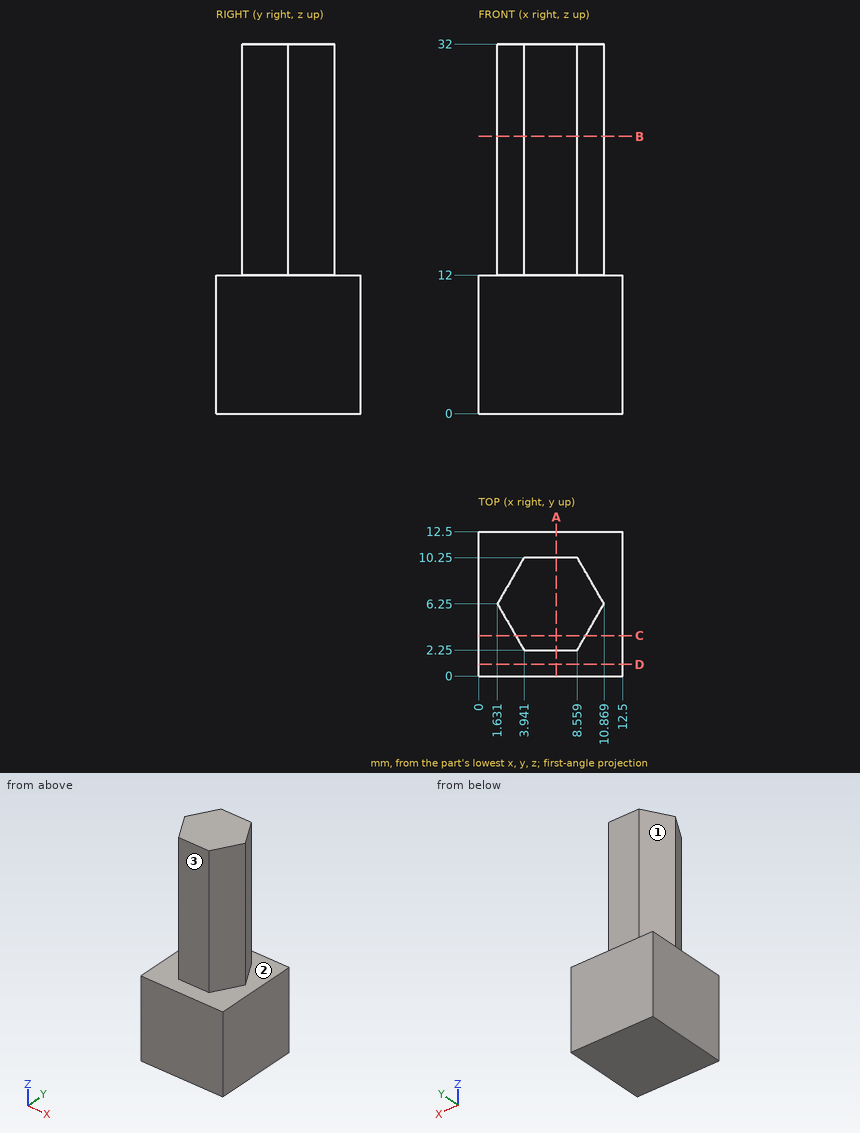
Could you check a few things on this drawing? It's one solid part, dimensions in mm from its lowest x, y, z. A direction names the side the tool comes from. Give positions to 0.01 mm unless a question says otherwise; leave off trailing zeros. Write each loop counter-clockwise with the first axis right and the second up, starting at its lowest first coordinate (ties: lowest second). Pieces come first, ordered by that corner, then holes. Notation, with made-up numbers: M 25.25,40.5 L 34.25,40.5 A23 cw 34.25,75.5 Z; hole C 27.25,-40 d1. An arc over 180 degrees is marked long. Put each result on its own line as item: value. Start each with the question number.
Item 1: If we section it at B-B, the plane z = 24: Write out the boundary of the cut face in (x, y), then the cut area to 3 significant figures.
Item 2: Will these pins go through, and if not, where does the flat tip stop? pin 1 (2.5 mm diameter, centred on x = 6, z = 26.5, fed in from -Y); pin 2 (1.4 mm diameter, centred on x = 5, z = 25, fed in from +Y); pin 3 (1.5 mm diameter, centred on y = 3.5, z = 18.5, fed in from -X) (1 decimal).
Item 3: If we section it at C-C, the plane y = 3.5: Write out the boundary of the cut face in (x, z).
Item 4: I need wall thicknesses on L1, parallel to Z at x = 3.5, y = 2.75; L2, parallel to Y at x = 5, z = 31; L3, parallel to X at y = 6.5, z = 25.5 (1 decimal). Which ranges of each line are inside material? Lowest first, please. Write a range as from..to.
Item 5: On a 3-axis mill with a long thin cutter (end or side, diameter ignored), from which of +Z, -Z, +X, -X, +Y, -Y can I reach the whole of each face in a straight line? I mean the marked faces 1, 2 and 3. Say none if no direction works.
Item 6: If we section it at A-A, the plane x = 6.75: Write out the boundary of the cut face in (y, z).
Item 7: If we section it at D-D, the plane y = 1: Write out the boundary of the cut face in (x, z), then the cut area to 3 significant figures.
Values:
1. outline: M 1.63,6.25 L 3.94,2.25 L 8.56,2.25 L 10.87,6.25 L 8.56,10.25 L 3.94,10.25 Z
1. area: 55.4 mm²
2. pin 1: y = 2.25
2. pin 2: y = 10.25
2. pin 3: x = 2.8
3. outline: M 0,0 L 12.5,0 L 12.5,12 L 9.28,12 L 9.28,32 L 3.22,32 L 3.22,12 L 0,12 Z
4. L1: 0..12
4. L2: 2.25..10.25
4. L3: 1.8..10.7
5. face 1: +Z, -X, +Y
5. face 2: +Z
5. face 3: +Z, +X, -X, -Y
6. outline: M 0,0 L 12.5,0 L 12.5,12 L 10.25,12 L 10.25,32 L 2.25,32 L 2.25,12 L 0,12 Z
7. outline: M 0,0 L 12.5,0 L 12.5,12 L 0,12 Z
7. area: 150 mm²
